Check sheet for the modelled part. Datum: model origin and axes. Units: mm. A direction names the side the tool comes from. Round coordinates to 2 decimals unless told otherwise and drop trailing zeros. Write each loop counter-clockwise with the first axis right and the second up, starting at its lowest first coordinate (ties: lowest second). Pieces come first, ordered by that corner, then holes. Notation, with made-up numbers: (18, 63) -> (43, 63) arc R21 ccw to (43, 97) -> close; hole circle Ø4 at (85.5, 21.5). An arc over 180 degrees is marked (long way). One line per item, written item: value.
Autodesk Inventor part; units mm, degrees
ref_plane "YZ Plane" through (0, 0, 0) normal (1, 0, 0) x (0, 1, 0)
ref_plane "XZ Plane" through (0, 0, 0) normal (0, 1, 0) x (-1, 0, 0)
ref_plane "XY Plane" through (0, 0, 0) normal (0, 0, 1) x (1, 0, 0)
sketch "Sketch1" plane through (0, 0, 0) normal (0, 1, 0) x (-1, 0, 0)
  line L0 (70, -46) -> (-70, -46)
  line L1 (-70, -46) -> (-70, 46)
  line L2 (-70, 46) -> (70, 46)
  line L3 (70, 46) -> (70, -46)
  point P0 (0, 0)
  point P1 (0, -46)
  point P2 (-70, 0)
  dimension "d0" = 140
  dimension "d1" = 92
extrude "Extrusion1" add sketch "Sketch1" along normal blind 4
sketch "Sketch2" plane through (0, 4, 0) normal (0, 1, 0) x (1, 0, 0)
  line L0 (70, 46) -> (-70, 46)
  line L1 (-70, 46) -> (-70, -46)
  line L2 (-70, -46) -> (70, -46)
  line L3 (70, -46) -> (70, 46)
  line L4 (-70, 46) -> (70, 46)
  line L5 (70, 46) -> (70, -46)
  line L6 (70, -46) -> (-70, -46)
  line L7 (-70, -46) -> (-70, 46)
  line L8 (-66, 42) -> (66, 42)
  line L9 (66, 42) -> (66, -42)
  line L10 (66, -42) -> (-66, -42)
  line L11 (-66, -42) -> (-66, 42)
  point P0 (0, 0)
  point P1 (0, -42)
  dimension "d4" = 4
  dimension "d5" = 4
  dimension "d6" = 4
  dimension "d7" = 4
extrude "Extrusion3" add sketch "Sketch2" along normal blind 38.1
sketch "Sketch3" plane through (0, 42.1, 0) normal (0, 1, 0) x (1, 0, 0)
  line L0 (66, 42) -> (66, -42)
  line L1 (66, -42) -> (-66, -42)
  line L2 (-66, -42) -> (-66, 42)
  line L3 (-66, 42) -> (66, 42)
  line L4 (70, 46) -> (-70, 46)
  line L5 (-70, 46) -> (-70, -46)
  line L6 (-70, -46) -> (70, -46)
  line L7 (70, -46) -> (70, 46)
  line L8 (-66, 42) -> (-66, -42)
  line L9 (-66, -42) -> (66, -42)
  line L10 (-66, 42) -> (-51, 42)
  line L11 (-51, 42) -> (-51, -42)
  line L12 (-51, -42) -> (-66, -42)
  line L13 (-66, -42) -> (-66, 42)
  line L14 (66, 42) -> (51, 42)
  line L15 (51, 42) -> (51, -42)
  line L16 (51, -42) -> (66, -42)
  line L17 (66, -42) -> (66, 42)
  point P0 (0, 0)
  dimension "d17" = 19
  dimension "d60" = 19
extrude "Extrusion4" add sketch "Sketch3" against normal blind 14 contours L0 L1 L15 L3 | L11 L1 L2 L3
sketch "Sketch5" plane through (70, 0, 46) normal (1, 0, 0) x (0, 0, -1)
  line L0 (92, 0) -> (0, 0)
  line L1 (92, 0) -> (92, 42.1)
  line L2 (0, 42.1) -> (92, 42.1)
  line L3 (0, 0) -> (0, 42.1)
  line L4 (92, 42.1) -> (0, 42.1)
  line L5 (19.15, 42.1) -> (27.15, 42.1)
  line L6 (27.15, 38.1) -> (30.15, 38.1)
  line L7 (30.15, 38.1) -> (30.15, 32.1)
  line L8 (30.15, 32.1) -> (16.15, 32.1)
  line L9 (16.15, 32.1) -> (16.15, 38.1)
  line L10 (16.15, 38.1) -> (19.15, 38.1)
  line L11 (19.15, 38.1) -> (19.15, 42.1)
  line L12 (27.15, 42.1) -> (27.15, 38.1)
  line L13 (64.85, 42.1) -> (72.85, 42.1)
  line L14 (72.85, 38.1) -> (75.85, 38.1)
  line L15 (75.85, 38.1) -> (75.85, 32.1)
  line L16 (75.85, 32.1) -> (61.85, 32.1)
  line L17 (61.85, 32.1) -> (61.85, 38.1)
  line L18 (61.85, 38.1) -> (64.85, 38.1)
  line L19 (64.85, 38.1) -> (64.85, 42.1)
  line L20 (72.85, 42.1) -> (72.85, 38.1)
  line L21 (0, 42.1) -> (92, 42.1)
  point P0 (46, 0)
  point P1 (23.15, 42.1)
  point P2 (23.15, 32.1)
  point P3 (68.85, 42.1)
  point P4 (68.85, 32.1)
  dimension "d47" = 14
  dimension "d48" = 6
  dimension "d49" = 8
  dimension "d50" = 10
  dimension "d51" = 23.15
  dimension "d52" = 14
  dimension "d53" = 6
  dimension "d54" = 8
  dimension "d56" = 10
  dimension "d57" = 23.15
extrude "Extrusion7" cut sketch "Sketch5" against normal blind 19 contours L20 L14 L15 L16 L17 L18 L19 L2 | L2 L12 L6 L7 L8 L9 L10 L11
sketch "Sketch6" plane through (-70, 0, -46) normal (-1, 0, 0) x (0, 0, 1)
  line L0 (92, 0) -> (0, 0)
  line L1 (92, 0) -> (92, 42.1)
  line L2 (0, 42.1) -> (92, 42.1)
  line L3 (0, 0) -> (0, 42.1)
  line L4 (64.85, 42.1) -> (72.85, 42.1)
  line L5 (72.85, 38.1) -> (75.85, 38.1)
  line L6 (75.85, 38.1) -> (75.85, 32.1)
  line L7 (75.85, 32.1) -> (61.85, 32.1)
  line L8 (61.85, 32.1) -> (61.85, 38.1)
  line L9 (61.85, 38.1) -> (64.85, 38.1)
  line L10 (64.85, 38.1) -> (64.85, 42.1)
  line L11 (72.85, 42.1) -> (72.85, 38.1)
  line L12 (19.15, 42.1) -> (27.15, 42.1)
  line L13 (27.15, 38.1) -> (30.15, 38.1)
  line L14 (30.15, 38.1) -> (30.15, 32.1)
  line L15 (30.15, 32.1) -> (16.15, 32.1)
  line L16 (16.15, 32.1) -> (16.15, 38.1)
  line L17 (16.15, 38.1) -> (19.15, 38.1)
  line L18 (19.15, 38.1) -> (19.15, 42.1)
  line L19 (27.15, 42.1) -> (27.15, 38.1)
  line L20 (0, 42.1) -> (92, 42.1)
  point P0 (46, 0)
  point P1 (68.85, 42.1)
  point P2 (68.85, 32.1)
  point P3 (23.15, 42.1)
  point P4 (23.15, 32.1)
  dimension "d61" = 14
  dimension "d62" = 6
  dimension "d63" = 8
  dimension "d65" = 14
  dimension "d66" = 6
  dimension "d67" = 8
  dimension "d69" = 10
  dimension "d70" = 23.15
  dimension "d71" = 23.15
  dimension "d72" = 10
extrude "Extrusion8" cut sketch "Sketch6" against normal blind 19 contours L11 L5 L6 L7 L8 L9 L10 L2 | L2 L19 L13 L14 L15 L16 L17 L18
sketch "Sketch7" plane through (0, 4, 0) normal (0, 1, 0) x (1, 0, 0)
  line L0 (66, -42) -> (66, 42)
  line L1 (66, 42) -> (-66, 42)
  line L2 (-66, 42) -> (-66, -42)
  line L3 (-66, -42) -> (66, -42)
  circle A0 centre (-16, 35) radius 3
  circle A1 centre (-16, -14) radius 3
  circle A2 centre (42, 35) radius 3
  circle A3 centre (42, -14) radius 3
  line L4 (-70, 26.85) -> (-51, 26.85)
  line L5 (-51, 26.85) -> (-51, 42)
  line L6 (-51, 42) -> (51, 42)
  line L7 (51, 42) -> (51, 26.85)
  line L8 (51, 26.85) -> (70, 26.85)
  line L9 (70, 26.85) -> (70, 46)
  line L10 (70, 46) -> (-70, 46)
  line L11 (-70, 46) -> (-70, 26.85)
  point P0 (0, 0)
  dimension "d75" = 6
  dimension "d76" = 6
  dimension "d77" = 49
  dimension "d78" = 58
  dimension "d79" = 6
  dimension "d80" = 6
  dimension "d82" = 7
  dimension "d92" = 35
extrude "Extrusion9" add sketch "Sketch7" along normal blind 6 contours A0 | A1 | A2 | A3
sketch "Sketch8" plane through (-16, 10, -35) normal (0, 1, 0) x (1, 0, 0)
  circle A0 centre (0, 0) radius 3
  circle A1 centre (0, -49) radius 3
  circle A2 centre (58, 0) radius 3
  circle A3 centre (58, -49) radius 3
  circle A4 centre (58, -49) radius 3
  circle A5 centre (0, 0) radius 3
  point P0 (16, -35)
hole "Hole1" at (-16, 10, -35) at (-16, 10, 14) at (42, 10, -35) at (42, 10, 14) direction (0, -1, 0) diameter 2.75 end through all
sketch "Sketch9" plane through (70, 0, -46) normal (0, 0, -1) x (-1, 0, 0)
  line L0 (19, 38.1) -> (19, 42.1)
  line L1 (19, 42.1) -> (19, 38.1)
  line L2 (19, 38.1) -> (19, 32.1)
  line L3 (19, 32.1) -> (19, 38.1)
  line L4 (19, 38.1) -> (19, 42.1)
  line L5 (19, 28.1) -> (19, 42.1)
  line L6 (19, 42.1) -> (19, 28.1)
  line L7 (19, 42.1) -> (19, 38.1)
  line L8 (19, 38.1) -> (19, 32.1)
  line L9 (19, 32.1) -> (19, 38.1)
  line L10 (121, 42.1) -> (121, 38.1)
  line L11 (121, 38.1) -> (121, 32.1)
  line L12 (121, 32.1) -> (121, 38.1)
  line L13 (121, 38.1) -> (121, 42.1)
  line L14 (121, 28.1) -> (121, 42.1)
  line L15 (121, 42.1) -> (121, 28.1)
  line L16 (121, 42.1) -> (121, 38.1)
  line L17 (121, 38.1) -> (121, 32.1)
  line L18 (121, 32.1) -> (121, 38.1)
  line L19 (121, 38.1) -> (121, 42.1)
  line L20 (19, 42.1) -> (121, 42.1)
  line L21 (121, 42.1) -> (121, 10)
  line L22 (121, 10) -> (19, 10)
  line L23 (19, 10) -> (19, 42.1)
  line L24 (89, 10) -> (83, 10)
  point P0 (70, 0)
extrude "Extrusion10" cut sketch "Sketch9" against normal up to surface (4 mm away)
sketch "Sketch10" plane through (0, 0, 0) normal (0, -1, 0) x (1, 0, 0)
  line L0 (44.3813, -32.6187) -> (39.6188, -32.6188)
  line L1 (39.6188, -32.6188) -> (39.6188, -37.3813)
  line L2 (39.6188, -37.3813) -> (44.3813, -37.3813)
  line L3 (44.3813, -37.3813) -> (44.3813, -32.6187)
  circle A0 centre (42, -35) radius 1.375
  circle A1 centre (42, -35) radius 1.375
  circle A2 centre (-16, -35) radius 1.375
  circle A3 centre (-16, 14) radius 1.375
  circle A4 centre (42, 14) radius 1.375
  line L4 (-70, -46) -> (70, -46)
  line L5 (70, -46) -> (70, 46)
  line L6 (70, 46) -> (-70, 46)
  line L7 (-70, 46) -> (-70, -46)
  line L8 (-13.6187, -37.3812) -> (-18.3812, -37.3812)
  line L9 (-18.3812, -37.3812) -> (-18.3812, -32.6187)
  line L10 (-18.3812, -32.6187) -> (-13.6187, -32.6188)
  line L11 (-13.6187, -32.6188) -> (-13.6187, -37.3812)
  line L12 (44.3813, 11.6188) -> (39.6188, 11.6188)
  line L13 (39.6188, 11.6188) -> (39.6188, 16.3813)
  line L14 (39.6188, 16.3813) -> (44.3813, 16.3813)
  line L15 (44.3813, 16.3813) -> (44.3813, 11.6188)
  line L16 (-13.6187, 11.6188) -> (-18.3812, 11.6188)
  line L17 (-18.3812, 11.6188) -> (-18.3812, 16.3813)
  line L18 (-18.3812, 16.3813) -> (-13.6187, 16.3813)
  line L19 (-13.6187, 16.3813) -> (-13.6187, 11.6188)
  point P0 (0, 0)
  point P1 (42, -32.6187)
  point P2 (39.6188, -35)
  point P3 (-18.3812, -35)
  point P4 (-18.3812, 14)
  point P5 (39.6188, 14)
  point P6 (-16, -37.3813)
  point P7 (-16, 11.6188)
  point P8 (42, 11.6188)
  dimension "d95" = 4.7625
  dimension "d96" = 4.7625
  dimension "d97" = 4.7625
  dimension "d98" = 4.7625
  dimension "d99" = 4.7625
  dimension "d100" = 4.7625
  dimension "d101" = 4.7625
  dimension "d102" = 4.7625
extrude "Extrusion11" cut sketch "Sketch10" against normal blind 1.5875 contours L3 L2 L1 L0 | L8 L9 L10 L11 | L12 L13 L14 L15 | L16 L17 L18 L19
sketch "Sketch11" plane through (0, 4, 0) normal (0, 1, 0) x (1, 0, 0)
  circle A0 centre (42, 35) radius 3
  circle A1 centre (-16, 35) radius 3
  circle A2 centre (-16, -14) radius 3
  circle A3 centre (42, -14) radius 3
  line L0 (66, -42) -> (66, 42)
  line L1 (66, 42) -> (-66, 42)
  line L2 (-66, 42) -> (-66, -42)
  line L3 (-66, -42) -> (66, -42)
  circle A4 centre (30.3953, -27.3279) radius 6.6721
  circle A5 centre (13, 10.5) radius 26.9638
  circle A6 centre (-27.6047, -27.3279) radius 6.6721
  circle A7 centre (-36.1, 10.5) radius 14.1362
  circle A8 centre (-51.3279, -27.3279) radius 6.6721
  circle A9 centre (52.9819, 10.5) radius 5.0181
  circle A10 centre (42, -14) radius 1.375 construction
  circle A11 centre (13, 10.5) radius 37.9638 construction
  circle A12 centre (-36.1, 10.5) radius 31.6901 construction
  point P0 (0, 0)
  point P1 (-66, 0)
  dimension "d105" = 8
  dimension "d106" = 8
  dimension "d107" = 8
  dimension "d108" = 8
  dimension "d109" = 8
  dimension "d110" = 8
  dimension "d112" = 8
  dimension "d113" = 8
  dimension "d114" = 8
  dimension "d115" = 8
  dimension "d116" = 8
extrude "Extrusion12" cut sketch "Sketch11" against normal through all contours A4 | A5 | A6 | A7 | A8 | A9
fillet "Fillet1" radius 2 38 edges at (51, 26.05, -46) (70, 21.05, -46) (0, 10, -46) (0, 10, -42) (-51, 26.05, -46) (-70, 21.05, -46) (-70, 21.05, 46) (66, 16.05, 42) (0, 4, 42) (66, 4, 0) (51, 19.05, -42) (51, 35.1, 42) (47.9638, 4, -10.5) (-13.9638, 4, -10.5) (23.7232, 4, 27.3279) (-51, 35.1, 42) (-51, 19.05, -42) (-66, 4, 0) (-66, 16.05, 42) (-66, 16.05, -42) (0, 4, -42) (-50.2362, 4, -10.5) (-58, 4, 27.3279) (-34.2768, 4, 27.3279) (66, 16.05, -42) (39, 4, 14) (-19, 4, 14) (39, 4, -35) (-19, 4, -35) (70, 21.05, 46) (-51, 28.1, 0) (51, 28.1, 0) (66, 28.1, 0) (-66, 28.1, 0) (-58.5, 28.1, 42) (58.5, 28.1, 42) (58.5, 28.1, -42) (-58.5, 28.1, -42)
ref_plane "Work Plane1" through (70, 0, -12.6625) normal (0, 0, -1) x (-1, 0, 0)
ref_plane "Work Plane2" through (30.3125, 0, 46) normal (1, 0, 0) x (0, 0, -1)
sketch "Sketch12" plane through (70, 0, -12.6625) normal (0, 0, -1) x (-1, 0, 0)
  line L0 (-7.5665, 44.2151) -> (155.3884, 44.2151)
  line L1 (155.3884, 44.2151) -> (155.3884, -4.8886)
  line L2 (155.3884, -4.8886) -> (-7.5665, -4.8886)
  line L3 (-7.5665, -4.8886) -> (-7.5665, 44.2151)
  point P0 (70, 0)
extrude "Extrusion13" cut sketch "Sketch12" against normal through all
sketch "Sketch13" plane through (30.3125, 0, 46) normal (1, 0, 0) x (0, 0, -1)
  line L0 (110.5301, 56.5997) -> (-15.9229, 56.5997)
  line L1 (-15.9229, 56.5997) -> (-15.9229, -18.7941)
  line L2 (-15.9229, -18.7941) -> (110.5301, -18.7941)
  line L3 (110.5301, -18.7941) -> (110.5301, 56.5997)
  point P0 (46, 0)
extrude "Extrusion14" cut sketch "Sketch13" against normal through all
equation "\"d5\" = d4"
equation "\"d6\" = d4"
equation "\"d7\" = d4"
equation "\"d60\" = d17"
equation "\"d56\" = d50"
equation "\"d69\" = d72"
equation "\"d76\" = d75"
equation "\"d79\" = d75"
equation "\"d80\" = d75"
equation "\"d96\" = d95"
equation "\"d97\" = d95"
equation "\"d98\" = d96"
equation "\"d99\" = d96"
equation "\"d100\" = d96"
equation "\"d101\" = d96"
equation "\"d102\" = d96"
equation "\"d106\" = d105"
equation "\"d107\" = d106"
equation "\"d108\" = d105"
equation "\"d110\" = d108"
equation "\"d112\" = d105"
equation "\"d113\" = d110"
equation "\"d114\" = d112"
equation "\"d115\" = d112"
equation "\"d116\" = d112"
properties part number "controlBox" material "ABS Plastic"
Item 1: Release check for a two-part mould opening along Y. For faces 5 (the flat face through (30.312, 3, -40)), 6 (the flat face through (60, 42.1, -37)), 7 (the flat face through (58, 28.1, -27)) record: pulls with the +Y half, pulls with the -Y half, needs draft (parallel to the pull), parting line crosses it, or undercut.
Result set:
face 5: needs draft
face 6: pulls with the +Y half
face 7: undercut
Item 2: Material ranges on line 1 along Z through (x, y) = (42, 8) (3 decimals); line 2 along X through (y, z) = (6, -35) (3 decimals); line 3 along Y through (x, z) = (53.5, -38), recorded low to high.
Result set:
line 1: -46 to -42, -38 to -36.375, -33.625 to -32
line 2: 39 to 40.625, 43.375 to 45, 66 to 70
line 3: 0 to 4, 28.1 to 42.1
Item 3: Sectioned sample at B-B (z = -35). Enter the section's corners in (x, y) (1 decimal), then the cut area to 3 significant figures.
Result set:
outline: (30.3, 0) -> (39.6, 0) -> (39.6, 1.6) -> (40.6, 1.6) -> (40.6, 10) -> (39, 10) -> (39, 6) arc R2 cw to (37, 4) -> (30.3, 4) -> close; (43.4, 1.6) -> (44.4, 1.6) -> (44.4, 0) -> (70, 0) -> (70, 42.1) -> (51, 42.1) -> (51, 30.1) arc R2 ccw to (53, 28.1) -> (64, 28.1) arc R2 cw to (66, 26.1) -> (66, 6) arc R2 cw to (64, 4) -> (47, 4) arc R2 cw to (45, 6) -> (45, 10) -> (43.4, 10) -> close
area: 529 mm^2
Item 4: Tool access check on faces 1 (the cylindrical face through (51.57, 17.18, -42.6)), 2 (the cylindrical face through (39.79, 7.97, -32.97)), 3 (the flat face through (61, 35, -29.85)), 4 (the flat face through (42, 1, -37.381)). Record the directions out of +Z, -Z, +X, -X, +Y, -Y that give a thin tool (end or side, any length) a straight path to the whole face; none if there is none.
Result set:
face 1: +Z, -X
face 2: +Y
face 3: +X, -X
face 4: -Y
Item 5: Sectioned sample at A-A (y = 37). Enter the section's corners in (x, z), then the cut area to 3 significant figures.
Result set:
outline: (51, -44) arc R2 ccw to (53, -46) -> (68, -46) arc R2 ccw to (70, -44) -> (70, -29.85) -> (51, -29.85) -> close; (51, -15.85) -> (70, -15.85) -> (70, -12.66) -> (51, -12.66) -> close
area: 366 mm^2
Item 6: Depth check by flat-ended pin: pin 1 (10 mm diameter, centred on y = 16, z = -27.5, fed in from -X); pin 2 (13.5 mm diameter, centred on x = 45.5, z = -32.5, fed in from +Y); pin 3 (2 mm diameter, centred on x = 43.5, z = -16.5, fed in from +Y); pin 4 (15.5 mm diameter, centred on y = 26.5, z = -23, fed in from -X). Enter the tip coordinate at first touch or a pass-through.
Result set:
pin 1: x = 66
pin 2: y = 42.1
pin 3: y = 4
pin 4: x = 51
